Part print with two shaded views. Sizes in mm from the minimum x, y, z corner. Coordinates: 2 decimals unless noted, no trailing zeros. Loops run counter-clockwise (first coordinate to the right, second up) from the corner with the lowest first, then second, coordinate; pieces in that order, holes last. Notation, with made-up numbers: (33, 55.25) - (63, 55.25) arc R10 cw to (63, 71.25) - close; hole circle Ø5 at (18.25, 39.5). An arc over 180 degrees is marked (long way). Answer as CSV lines item,"result".
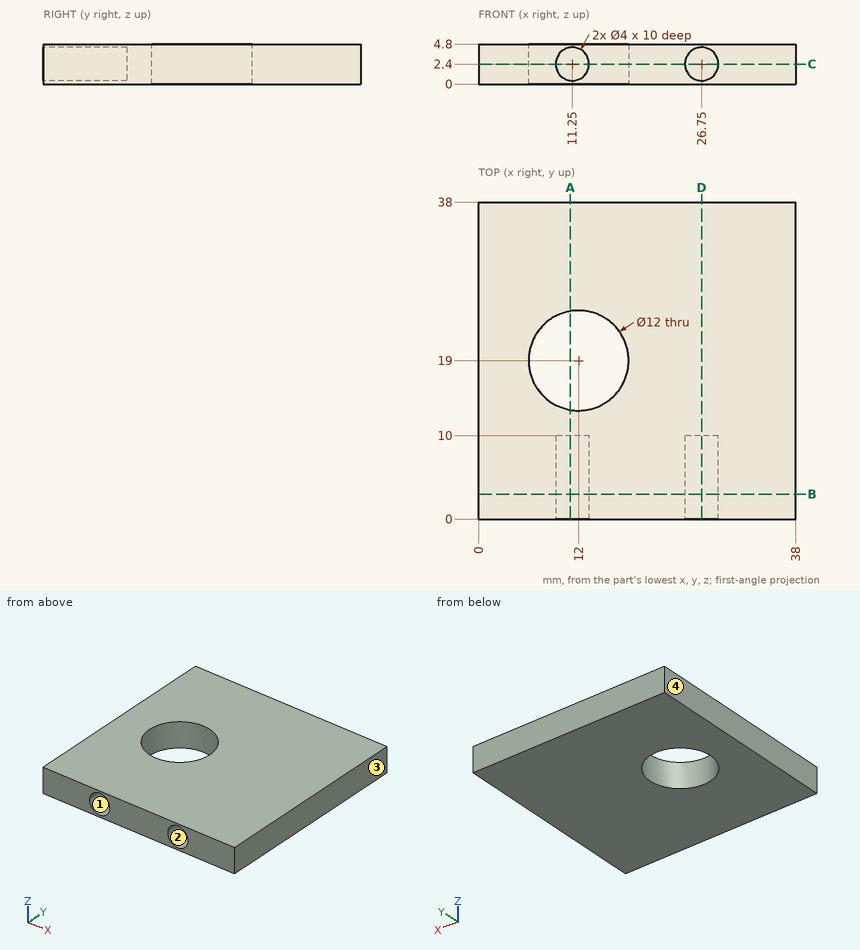
Q1. Saw through at B-B (y = 3). Give the cut face in (x, z), then the cut area to 3 significant figures.
Results:
outline,"(0, 0) - (38, 0) - (38, 4.8) - (0, 4.8) - close; hole circle Ø4 at (11.25, 2.4); hole circle Ø4 at (26.75, 2.4)"
area,"157 mm^2"
Q2. Saw through at D-D (x = 26.75). Give the cut face in (y, z).
Results:
outline,"(0, 0) - (38, 0) - (38, 4.8) - (0, 4.8) - (0, 4.4) - (10, 4.4) - (10, 0.4) - (0, 0.4) - close"
Q3. Wall check: L1, parallel to Z at x = 11.25, y = 5.25; L2, parallel to X at y = 9.5, z = 2.9; L3, parallel to Y at x = 12, z = 3.45. Give the ranges that are in metal, low to high.
Results:
L1,"z = 0 to 0.4, 4.4 to 4.8"
L2,"x = 0 to 9.31, 13.19 to 24.81, 28.69 to 38"
L3,"y = 10 to 13, 25 to 38"
Q4. Saw through at A-A (x = 11). Give the cut face in (y, z).
Results:
outline,"(0, 0) - (13.08, 0) - (13.08, 4.8) - (0, 4.8) - (0, 4.38) - (10, 4.38) - (10, 0.42) - (0, 0.42) - close; (24.92, 0) - (38, 0) - (38, 4.8) - (24.92, 4.8) - close"
Q5. Flat gauge pin, fed straight in: pin 1 (2 mm diameter, centred on x = 11.5, z = 3, fed in from -Y). Where does the tip first touch, or does it go through?
Results:
pin 1,"stops at y = 10"
Q6. Saw through at C-C (z = 2.4). Give the cut face in (x, y), then the cut area to 3 significant figures.
Results:
outline,"(0, 0) - (9.25, 0) - (9.25, 10) - (13.25, 10) - (13.25, 0) - (24.75, 0) - (24.75, 10) - (28.75, 10) - (28.75, 0) - (38, 0) - (38, 38) - (0, 38) - close; hole circle Ø12 at (12, 19)"
area,"1,250 mm^2"
Q7. Two-plate mould, pull along X, no slides. Class the marked faces 1, 2, 3 and 4: released by +X, released by -X, zero draft, split by the parting line, or undercut.
Results:
face 1,"undercut"
face 2,"undercut"
face 3,"released by +X"
face 4,"released by -X"
